from build123d import *

# Parameters (mm, degrees)
SKETCH1_W           = 50
SKETCH1_H           = 85
BOSS_EXTRUDE1_DEPTH = 38.5
M5_TAPPED_HOLE1_D   = 4.2
SKETCH6_R           = 14
CUT_EXTRUDE1_DEPTH  = 86
SKETCH8_R           = 14
SKETCH8_R_2         = 8
BOSS_EXTRUDE2_DEPTH = 39


with BuildPart() as part:
    # Sketch1 → Boss-Extrude1 (new body)
    with BuildSketch(Plane.XY):
        Rectangle(SKETCH1_W, SKETCH1_H)
    extrude(amount=BOSS_EXTRUDE1_DEPTH)

    # M5 Tapped Hole1 (through all)
    with Locations(Plane.XY.offset(38.5)):
        with Locations((-18, 30), (18, 30), (18, -30), (-18, -30)):
            Hole(M5_TAPPED_HOLE1_D / 2)

    # Sketch6 → Cut-Extrude1 (cut, through all)
    with BuildSketch(Plane(origin=(0, 42.5, 0), x_dir=(1, 0, 0), z_dir=(0, 1, 0))):
        with Locations((0, -19.5)):
            Circle(SKETCH6_R)
        Polygon((-25, -10.5), (-14.5, 0), (-25, 0), align=None)
        Polygon((25, -10.5), (14.5, 0), (25, 0), align=None)
    extrude(amount=-CUT_EXTRUDE1_DEPTH, mode=Mode.SUBTRACT)

    # Sketch8 → Boss-Extrude2 (add, symmetric)
    with BuildSketch(Plane(origin=(0, 0, 0), x_dir=(-1, 0, 0), z_dir=(0, -1, 0))):
        with Locations((0, -19.5)):
            Circle(SKETCH8_R)
        with Locations((0, -19.5)):
            Circle(SKETCH8_R_2, mode=Mode.SUBTRACT)
    extrude(amount=BOSS_EXTRUDE2_DEPTH, both=True)


solid = part.part
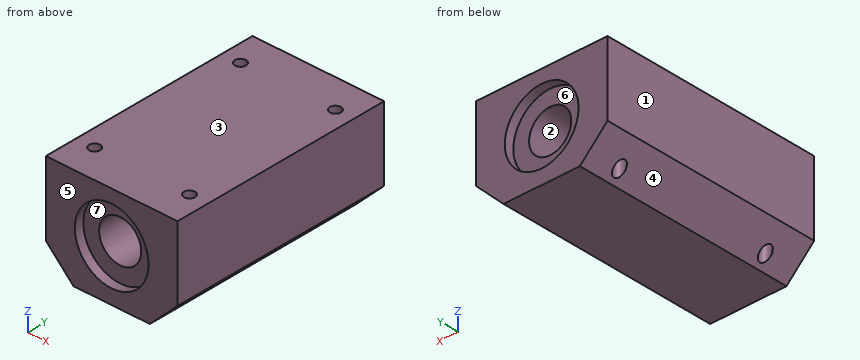
The listing builds one solid part. Answer for the finished solid, in the listing's coordinates (mm). Face numbers are marked on the shaded views. A direction names the side the tool comes from. Give positions to 0.01 mm unless a question says otherwise; leave off trailing zeros. Order: outer loops, then holes, each group sorted by start corner. A loop starts at its lowest first (then second) coordinate and runs counter-clockwise, first axis right, second up. Notation, with made-up numbers: (-2.5, 58.25) -> (21.5, 58.25) arc R8 ccw to (21.5, 73.25) -> close; hole circle Ø10 at (61.25, 28.5). An arc over 180 degrees is marked (long way). Put each result on its own line as item: value.
Item 1: Given P1, Ø17, axis at x = 0, z = 19.5, coming from the -Y side; P2, Ø4, axis at x = -18, y = 30, coming from the -Z side; P3, Ø5, axis at x = -5, z = 22, coming from the +Y side; P4, Ø1.5, axis at y = -15, z = 4, coming from the -X side, each flat-ended and moving along its own axis, determine where each tip first touches the part or whether it passes through.
Established:
P1: stops at y = -39
P2: passes through
P3: stops at y = 39
P4: stops at x = -19.25
Item 2: A cutting plane is placed at C-C on x = -18. Give the vertices of the cut face in (y, z).
Established:
outline: (-42.5, 3.5) -> (-32.1, 3.5) -> (-32.1, 38.5) -> (-42.5, 38.5) -> close; (-27.9, 3.5) -> (27.9, 3.5) -> (27.9, 38.5) -> (-27.9, 38.5) -> close; (32.1, 3.5) -> (42.5, 3.5) -> (42.5, 38.5) -> (32.1, 38.5) -> close
Item 3: For a pull along Z with two mould halves and no side action, classify the marked faces 1, 2, 3 and 4 as released by +Z, released by -Z, zero draft, split by the parting line, or undercut.
Established:
face 1: zero draft
face 2: undercut
face 3: released by +Z
face 4: released by -Z
Item 4: Straight lines are drawn through the part: line 1 (Y direction, x = -18, z = 23.5); line 2 (X direction, y = -30, z = 11); line 3 (Z direction, x = 0, y = -41). For each, find the intervals that lie inside material, in ascending order.
Established:
line 1: y = -42.5 to -32.1, -27.9 to 27.9, 32.1 to 42.5
line 2: x = -25 to -20.1, -15.9 to 15.9, 20.1 to 25
line 3: z = 0 to 5.5, 33.5 to 38.5
Item 5: A cutting plane is placed at A-A on y = -30. Give the vertices of the cut face in (x, z), plus the area to 3 significant figures.
Established:
outline: (-25, 10.5) -> (-20.1, 5.6) -> (-20.1, 38.5) -> (-25, 38.5) -> close; (-15.9, 1.4) -> (-14.5, 0) -> (14.5, 0) -> (15.9, 1.4) -> (15.9, 38.5) -> (-15.9, 38.5) -> close; (20.1, 5.6) -> (25, 10.5) -> (25, 38.5) -> (20.1, 38.5) -> close; hole circle Ø16 at (0, 19.5)
area: 1,320 mm^2
Item 6: A cutting plane is placed at D-D on x = 0. Give the vertices of the cut face in (y, z).
Established:
outline: (-42.5, 0) -> (42.5, 0) -> (42.5, 5.5) -> (39, 5.5) -> (39, 11.5) -> (-39, 11.5) -> (-39, 5.5) -> (-42.5, 5.5) -> close; (-42.5, 33.5) -> (-39, 33.5) -> (-39, 27.5) -> (39, 27.5) -> (39, 33.5) -> (42.5, 33.5) -> (42.5, 38.5) -> (-42.5, 38.5) -> close
Item 7: For the marked faces 5, 6 and 7, determine the directions among +Z, -Z, +X, -X, +Y, -Y from which every point of the face is accessible in a straight line to the end or side of a thin tool.
Established:
face 5: +Z, -Z, +X, -X, -Y
face 6: +Y
face 7: -Y
Item 8: A cutting plane is placed at B-B on z = 19.5. Give the vertices of the cut face in (x, y), plus the area to 3 significant figures.
Established:
outline: (-25, -42.5) -> (-14, -42.5) -> (-14, -39) -> (-8, -39) -> (-8, 39) -> (-14, 39) -> (-14, 42.5) -> (-25, 42.5) -> close; (8, -39) -> (14, -39) -> (14, -42.5) -> (25, -42.5) -> (25, 42.5) -> (14, 42.5) -> (14, 39) -> (8, 39) -> close; hole circle Ø4.2 at (-18, -30); hole circle Ø4.2 at (-18, 30); hole circle Ø4.2 at (18, -30); hole circle Ø4.2 at (18, 30)
area: 2,750 mm^2
